from build123d import *

# Parameters (mm, degrees)
F0_W     = 4.7625
F0_H     = 32.54375
F1_DEPTH = 4.7625
F3_DEPTH = 3.175
F4_DEPTH = 1.5875
F5_R     = 0.396875
F6_DEPTH = 32.54475


with BuildPart() as f1:
    # F0 (on Top) → F1 (new body)
    with BuildSketch(Plane.XY):
        Rectangle(F0_W, F0_H)
    extrude(amount=F1_DEPTH)

    # F2 (on face) → F3 (cut)
    with BuildSketch(Plane(origin=(0, 0, 0), x_dir=(1, 0, 0), z_dir=(0, 0, -1))):
        Polygon((2.38125, -16.271875), (2.38125, 14.684375), (-2.38125, 14.684375), (-2.38125, -16.271875), (-1.5875, -16.271875), (-1.5875, -14.684375), (1.5875, -14.684375), (1.5875, -16.271875), align=None)
    extrude(amount=-F3_DEPTH, mode=Mode.SUBTRACT)

    # F4 (cut): a face of the model
    f4_faces = [f1.faces().sort_by_distance(p)[0] for p in [
        (0, 15.478125, 0),
    ]]
    extrude(f4_faces, amount=-F4_DEPTH, mode=Mode.SUBTRACT)

    # F5 (on face) → F6 (cut, through all)
    with BuildSketch(Plane(origin=(0, 16.271875, 0), x_dir=(-1, 0, 0), z_dir=(0, 1, 0))):
        with Locations((0, 2.38125)):
            Circle(F5_R)
    extrude(amount=-F6_DEPTH, mode=Mode.SUBTRACT)


solid = f1.part
Verification items for the finished model (mm, model axes). A direction names the side the tool comes from. Coordinates: 2 decimals unless noted, no trailing zeros. Write each loop counter-clockwise with the first axis right and the second up, starting at its lowest first coordinate (ties: lowest second). Pieces come first, ordered by that corner, then holes. Notation, with made-up numbers: M -23,8.25 L 32,8.25 A33 cw 32,40.25 Z; hole C 18.25,77.25 d5. An arc over 180 degrees is marked long. Use CSV: the item, a comma, the result in double quotes.
Q1. Mould release check, pull along Y, two halves, no side actions. Record for faces 4 (the flat face through (0, 15, 1.588)), 5 (the flat face through (0, 16.272, 4)), 6 (the flat face through (0, 14.684, 3)), 7 (the flat face through (0, -14.684, 1.6)): pulls with the +Y half, pulls with the -Y half, needs draft (parallel to the pull), parting line crosses it, or undercut.
Computed values:
face 4,"needs draft"
face 5,"pulls with the +Y half"
face 6,"undercut"
face 7,"undercut"
Q2. Go/stop test with flat-tipped pins: P1, Ø2.5, axis at x = 1, z = 1, coming from the +Y side; P2, Ø2, axis at x = 0.5, y = -3, coming from the -Z side (3 decimals); P3, Ø0.5, axis at y = 16, z = 2.5, coming from the +X side; P4, Ø0.8, axis at x = -0.5, y = 15.5, coming from the -Z side. Record where each tip stops, or that it passes through.
Computed values:
P1,"y = 16.27"
P2,"z = 3.175"
P3,"x = 1.59"
P4,"z = 1.59"
Q3. Section check B-B, the plane z = 1. Enter the section's corners in (x, y), and give its area (3 significant figures).
Computed values:
outline,"M -2.38,-16.27 L 2.38,-16.27 L 2.38,-14.68 L -2.38,-14.68 Z"
area,"7.56 mm²"
Q4. Thickness scan on line 1 along Z through (x, y) = (0.05, -15); line 2 along Y through (x, z) = (-1.5, 2.15); line 3 along Z through (x, y) = (0, 15.4). Record the ranges inside material, lowest first. Write a range as [from, to].
Computed values:
line 1,"[0, 1.99], [2.77, 4.76]"
line 2,"[-16.27, -14.68], [14.68, 16.27]"
line 3,"[1.59, 1.98], [2.78, 4.76]"
Q5. Set-up check for faces 1 (the flat face through (-2.381, -3.8, 3.4)), 2 (the flat face through (1.588, 15, 2)), 3 (the flat face through (-1.588, 15, 2)): record each of +Z, -Z, +X, -X, +Y, -Y from which the full face is reachable in a straight line by a thin tool's end or side.
Computed values:
face 1,"+Z, -Z, -X, +Y, -Y"
face 2,"-Z, +X, +Y"
face 3,"-Z, -X, +Y"
Q6. Section check A-A, the plane x = 0. State how many separate pieces and enclosed holes the cut face has, and give its area (3 significant figures).
Computed values:
separate pieces,"3"
enclosed holes,"0"
area,"56.7 mm²"
Q7. Section check C-C, the plane y = -9. Enter the section's corners in (x, z) (1 decimal), and give its area (3 significant figures).
Computed values:
outline,"M -2.4,3.2 L 2.4,3.2 L 2.4,4.8 L -2.4,4.8 Z"
area,"7.56 mm²"
